Model file for the job. Use its own axes, mm. A direction names the side the tool comes from. Coordinates: 2 decimals unless noted, no trailing zeros. Order: outer loops, then holes, each group sorted by start corner. A loop starts at its lowest first (then second) coordinate and runs counter-clockwise, first axis right, second up. Notation, with made-up numbers: M 34.25,-25 L 68.25,-25 A21 cw 68.25,-13 Z; hole C 27.5,65.5 d7. An arc over 180 degrees is marked long. Return JSON: item names as keys, results as strings.
```python
from build123d import *

# Parameters (mm, degrees)
SKETCH_1_W      = 12.6
SKETCH_1_H      = 55
SKETCH_1_R      = 2.6
EXTRUDE_1_DEPTH = 5
SKETCH_2_R      = 4
EXTRUDE_2_DEPTH = 5


with BuildPart() as part:
    # 草图1 → 凸台-拉伸1 (new body)
    with BuildSketch(Plane(origin=(0, 0, 0), x_dir=(1, 0, 0), z_dir=(0, 1, 0))):
        Rectangle(SKETCH_1_W, SKETCH_1_H)
        with Locations(Location((0, 21, 0), (0, 0, 270))):
            Circle(SKETCH_1_R, mode=Mode.SUBTRACT)
        with Locations(Location((0, -21, 0), (0, 0, 270))):
            Circle(SKETCH_1_R, mode=Mode.SUBTRACT)
    extrude(amount=EXTRUDE_1_DEPTH)

    # 草图2 → 凸台-拉伸2 (add, symmetric)
    with BuildSketch(Plane(origin=(0, 0, 0), x_dir=(0, 0, -1), z_dir=(1, 0, 0))):
        with BuildLine():
            Line((-16, 5), (-14.921975395, 15.527956257))
            ThreePointArc((-14.921975395, 15.527956257), (0, 29), (14.921975395, 15.527956257))
            Line((14.921975395, 15.527956257), (16, 5))
            Line((16, 5), (-16, 5))
        make_face()
        with Locations((0, 14)):
            Circle(SKETCH_2_R, mode=Mode.SUBTRACT)
    extrude(amount=EXTRUDE_2_DEPTH, both=True)


solid = part.part
```
Item 1: Saw through at B-B (z = -21). Write the cut outline in (x, y).
Check result:
{"outline": "M -6.3,0 L -2.6,0 L -2.6,5 L -6.3,5 Z; M 2.6,0 L 6.3,0 L 6.3,5 L 2.6,5 Z"}
Item 2: Saw through at D-D (x = 3.25). Write the cut outline in (y, z).
Check result:
{"outline": "M 0,-27.5 L 5,-27.5 L 5,-16 L 15.53,-14.92 A15 ccw 15.53,14.92 L 5,16 L 5,27.5 L 0,27.5 Z; hole C 14,0 d8"}
Item 3: Pull direction Z, two halves, no side cores. Call faces 4 (the flat face through (0, 2, 27.5)), 5 (the cylindrical face through (0.78, 2.46, -18.52)), 6 (the flat face through (0.07, 10.338, -15.453)): +Z half, -Z half, draft (parallel to the pull), parting line (faces both ways), or undercut.
Check result:
{"face 4": "+Z half", "face 5": "undercut", "face 6": "-Z half"}
Item 4: Wall check: line 1 (X direction, y = 2.1, z = -21); line 2 (X direction, y = 17.25, z = 13.5); line 3 (Y direction, x = -3.25, z = -21). Give the ranges that are in metal, low to high.
Check result:
{"line 1": "x = -6.3 to -2.6, 2.6 to 6.3", "line 2": "x = -5 to 5", "line 3": "y = 0 to 5"}
Item 5: 3-axis set-ups, long thin cutter, end or side, ignore diameter. For faces 1 (the cylindrical face through (-0.07, 17.966, 0.521)), 2 (the flat face through (5, 17, -4)), 3 (the flat face through (-5, 17, -4)): which of +Z, -Z, +X, -X, +Y, -Y reach the whole face in a straight line?
Check result:
{"face 1": "+X, -X", "face 2": "+Z, -Z, +X, +Y", "face 3": "+Z, -Z, -X, +Y"}
Item 6: Saw through at C-C (y = 14). Write the cut outline in (x, z).
Check result:
{"outline": "M -5,-15.08 L 5,-15.08 L 5,-4 L -5,-4 Z; M -5,4 L 5,4 L 5,15.08 L -5,15.08 Z"}
Item 7: Drop flat-ended pins along their axis: pin 1 Ø6 at (x, z) = (0, 21) entering from +Y; pin 2 Ø3 at (x, y) = (3.5, 24.5) entering from +Z; pin 3 Ø10 at (y, z) = (12.5, 22) entering from +X; pin 4 Ø12 at (y, z) = (22, 4.5) entering from +X. Give the stop position or say it passes through.
Check result:
{"pin 1": "stops at y = 5", "pin 2": "stops at z = 12", "pin 3": "passes through", "pin 4": "stops at x = 5"}
Item 8: Saw through at A-A (x = 0). Write the cut outline in (y, z).
Check result:
{"outline": "M 0,-27.5 L 5,-27.5 L 5,-23.6 L 0,-23.6 Z; M 0,-18.4 L 5,-18.4 L 5,-16 L 15.53,-14.92 A15 ccw 15.53,14.92 L 5,16 L 5,18.4 L 0,18.4 Z; M 0,23.6 L 5,23.6 L 5,27.5 L 0,27.5 Z; hole C 14,0 d8"}
